Geometry: final body of the model. Coordinates: model frame, mm. A direction names the side the tool comes from. Round coordinates to 2 decimals unless told otherwise and drop trailing zeros. Loops run counter-clockwise (first coordinate to the right, second up) from the corner with the lowest first, then second, coordinate; pieces in that order, holes last. Notation, with made-up numbers: (19, -22) - (78, -22) arc R14 cw to (78, -13) - close; hole circle Ø10 at (4.25, 78.25). An arc over 180 degrees is marked (long way). Write item = value, one per line. Start each with the question number.
Item 1: Draft query along Z for faces 4 (the flat face through (0, 1, -27.403)), 5 (the cylindrical face through (-0.18, 4.02, 12.76)), 6 (the flat face through (-29.905, 4, 25)). Return one class per face: pulls with the +Z half, pulls with the -Z half, needs draft (parallel to the pull), parting line crosses it, or undercut.
Item 2: Section C-C (y = 1.05). Return loops of the section in (x, z), plus the area to 3 significant figures.
Item 3: Section A-A (x = 0). Return loops of the section in (y, z), plus the area to 3 significant figures.
Item 4: Section B-B (z = -22). Return loops of the section in (x, y).
Item 5: Section D-D (z = 9.5). Return loops of the section in (x, y).
Item 6: First-contact query: pin 1 (4 mm diameter, centred on x = -25.91, z = 24.6, fed in from -Y); pin 2 (1.1 mm diameter, centred on x = -29.5, y = 3, fed in from -Z); pin 3 (1.6 mm diameter, centred on x = -10, y = 0.5, fed in from +Z). Flat tips, straight axial feed; report the tip coordinate or a pass-through.
Item 7: Line query: line 1 (Z direction, x = 26, y = 3.45); line 2 (Z direction, x = 12, y = 3.1); line 3 (Z direction, x = -11, y = 4.9). Output: solid intervals per line, ascending. Write a range as from..to.
Item 8: Access query for faces 1 (the flat face through (-11.905, 5, -24)), 2 (the flat face through (0, 2, -33)), 3 (the flat face through (0, 2, 26)). Directions: +Z, -Z, +X, -X, +Y, -Y. A direction counts if a zero-diameter tool reaches every point of the face in a straight line with its end or side. Return the directions, or none.
from build123d import *

# Parameters (mm, degrees)
SKETCH1_W           = 60
SKETCH1_H           = 48
BOSS_EXTRUDE1_DEPTH = 2
BOSS_EXTRUDE2_DEPTH = 3.5
SKETCH3_W           = 6.52386431
SKETCH3_H           = 49
SKETCH3_W_2         = 6.523864309
CUT_EXTRUDE2_DEPTH  = 15
SKETCH4_W           = 24
SKETCH4_H           = 12
CUT_EXTRUDE3_DEPTH  = 1.5
SKETCH5_R           = 1.35
CUT_EXTRUDE4_DEPTH  = 3
SKETCH6_R           = 1.35
CUT_EXTRUDE5_DEPTH  = 3
SKETCH7_W           = 69.929961246
SKETCH7_H           = 12.314710156
SKETCH7_W_2         = 77.406749556
SKETCH7_H_2         = 16.199708004
CUT_EXTRUDE6_DEPTH  = 2
SKETCH8_R           = 1.6
CUT_EXTRUDE7_DEPTH  = 18
SKETCH9_W           = 6.597166155
SKETCH9_H           = 6.303958771
SKETCH9_W_2         = 5.93744954
SKETCH9_H_2         = 5.497638462
SKETCH9_W_3         = 7.769995694
SKETCH9_W_4         = 5.131129232
SKETCH9_H_3         = 5.204431078
SKETCH9_W_5         = 5.497638463
SKETCH9_H_4         = 5.0930957
SKETCH9_W_6         = 4.691318155
BOSS_EXTRUDE3_DEPTH = 3.5
SKETCH10_W          = 13.673673514
SKETCH10_H          = 2.686711401
SKETCH10_W_2        = 10.911645047
SKETCH10_H_2        = 3.141048784
SKETCH10_W_3        = 10.921694408
SKETCH10_H_3        = 3.054325349
SKETCH10_W_4        = 12
BOSS_EXTRUDE4_DEPTH = 3.5


with BuildPart() as part:
    # Sketch1 → Boss-Extrude1 (new body)
    with BuildSketch(Plane(origin=(0, 0, 0), x_dir=(1, 0, 0), z_dir=(0, 1, 0))):
        with Locations((0.094538135, 3.403372847)):
            Rectangle(SKETCH1_W, SKETCH1_H)
        with BuildLine():
            Line((-29.905461865, -20.596627153), (-29.905461865, -28.096627153))
            ThreePointArc((-29.905461865, -28.096627153), (-29.026782209, -30.217947496), (-26.905461865, -31.096627153))
            Line((-26.905461865, -31.096627153), (-24.905461865, -31.096627153))
            Line((-24.905461865, -31.096627153), (-24.905461865, -29.096627153))
            Line((-24.905461865, -29.096627153), (-14.905461865, -29.096627153))
            Line((-14.905461865, -29.096627153), (-14.905461865, -31.096627153))
            Line((-14.905461865, -31.096627153), (13.094538135, -31.096627153))
            Line((13.094538135, -31.096627153), (13.094538135, -29.096627153))
            Line((13.094538135, -29.096627153), (23.094538135, -29.096627153))
            Line((23.094538135, -29.096627153), (23.094538135, -31.096627153))
            Line((23.094538135, -31.096627153), (27.094538135, -31.096627153))
            ThreePointArc((27.094538135, -31.096627153), (29.215858478, -30.217947496), (30.094538135, -28.096627153))
            Line((30.094538135, -28.096627153), (30.094538135, -20.596627153))
            Line((30.094538135, -20.596627153), (-29.905461865, -20.596627153))
        make_face()
        with BuildLine():
            Line((30.094538135, 27.403372847), (30.094538135, 34.903372847))
            ThreePointArc((30.094538135, 34.903372847), (29.215858478, 37.024693191), (27.094538135, 37.903372847))
            Line((27.094538135, 37.903372847), (25.094538135, 37.903372847))
            Line((25.094538135, 37.903372847), (25.094538135, 35.903372847))
            Line((25.094538135, 35.903372847), (15.094538135, 35.903372847))
            Line((15.094538135, 35.903372847), (15.094538135, 37.903372847))
            Line((15.094538135, 37.903372847), (-12.905461865, 37.903372847))
            Line((-12.905461865, 37.903372847), (-12.905461865, 35.903372847))
            Line((-12.905461865, 35.903372847), (-22.905461865, 35.903372847))
            Line((-22.905461865, 35.903372847), (-22.905461865, 37.903372847))
            Line((-22.905461865, 37.903372847), (-26.905461865, 37.903372847))
            ThreePointArc((-26.905461865, 37.903372847), (-29.026782209, 37.024693191), (-29.905461865, 34.903372847))
            Line((-29.905461865, 34.903372847), (-29.905461865, 27.403372847))
            Line((-29.905461865, 27.403372847), (30.094538135, 27.403372847))
        make_face()
    extrude(amount=BOSS_EXTRUDE1_DEPTH)

    # Sketch2 → Boss-Extrude2 (add)
    with BuildSketch(Plane(origin=(0, 2, 0), x_dir=(1, 0, 0), z_dir=(0, 1, 0))):
        with BuildLine():
            Line((30.094538135, -11.096627153), (-29.905461865, -11.096627153))
            Line((-29.905461865, -11.096627153), (-29.905461865, -28.096627153))
            ThreePointArc((-29.905461865, -28.096627153), (-29.026782209, -30.217947496), (-26.905461865, -31.096627153))
            Line((-26.905461865, -31.096627153), (-24.905461865, -31.096627153))
            Line((-24.905461865, -31.096627153), (-24.905461865, -29.096627153))
            Line((-24.905461865, -29.096627153), (-14.905461865, -29.096627153))
            Line((-14.905461865, -29.096627153), (-14.905461865, -31.096627153))
            Line((-14.905461865, -31.096627153), (13.094538135, -31.096627153))
            Line((13.094538135, -31.096627153), (13.094538135, -29.096627153))
            Line((13.094538135, -29.096627153), (23.094538135, -29.096627153))
            Line((23.094538135, -29.096627153), (23.094538135, -31.096627153))
            Line((23.094538135, -31.096627153), (27.094538135, -31.096627153))
            ThreePointArc((27.094538135, -31.096627153), (29.215858478, -30.217947496), (30.094538135, -28.096627153))
            Line((30.094538135, -28.096627153), (30.094538135, -11.096627153))
        make_face()
        with BuildLine():
            Line((-29.905461865, 34.903372847), (-29.905461865, 17.903372847))
            Line((-29.905461865, 17.903372847), (30.094538135, 17.903372847))
            Line((30.094538135, 17.903372847), (30.094538135, 34.903372847))
            ThreePointArc((30.094538135, 34.903372847), (29.215858478, 37.024693191), (27.094538135, 37.903372847))
            Line((27.094538135, 37.903372847), (25.094538135, 37.903372847))
            Line((25.094538135, 37.903372847), (25.094538135, 35.903372847))
            Line((25.094538135, 35.903372847), (15.094538135, 35.903372847))
            Line((15.094538135, 35.903372847), (15.094538135, 37.903372847))
            Line((15.094538135, 37.903372847), (-12.905461865, 37.903372847))
            Line((-12.905461865, 37.903372847), (-12.905461865, 35.903372847))
            Line((-12.905461865, 35.903372847), (-22.905461865, 35.903372847))
            Line((-22.905461865, 35.903372847), (-22.905461865, 37.903372847))
            Line((-22.905461865, 37.903372847), (-26.905461865, 37.903372847))
            ThreePointArc((-26.905461865, 37.903372847), (-29.026782209, 37.024693191), (-29.905461865, 34.903372847))
        make_face()
    extrude(amount=BOSS_EXTRUDE2_DEPTH)

    # Sketch3 → Cut-Extrude2 (cut)
    with BuildSketch(Plane(origin=(0, 5.5, 0), x_dir=(1, 0, 0), z_dir=(0, 1, 0))):
        with Locations((-32.16739402, 3.403372847)):
            Rectangle(SKETCH3_W, SKETCH3_H)
        with Locations((32.35647029, 3.403372847)):
            Rectangle(SKETCH3_W_2, SKETCH3_H)
    extrude(amount=-CUT_EXTRUDE2_DEPTH, mode=Mode.SUBTRACT)

    # Sketch4 → Cut-Extrude3 (cut)
    with BuildSketch(Plane(origin=(0, 5.5, 0), x_dir=(1, 0, 0), z_dir=(0, 1, 0))):
        with Locations((0.094538135, 23.903372847)):
            Rectangle(SKETCH4_W, SKETCH4_H)
    extrude(amount=-CUT_EXTRUDE3_DEPTH, mode=Mode.SUBTRACT)

    # Sketch5 → Cut-Extrude4 (cut)
    with BuildSketch(Plane(origin=(0, 5.5, 0), x_dir=(1, 0, 0), z_dir=(0, 1, 0))):
        with Locations((0, -14.096627153)):
            Circle(SKETCH5_R)
    extrude(amount=-CUT_EXTRUDE4_DEPTH, mode=Mode.SUBTRACT)

    # Sketch6 → Cut-Extrude5 (cut)
    with BuildSketch(Plane(origin=(0, 5.5, 0), x_dir=(1, 0, 0), z_dir=(0, 1, 0))):
        with Locations((20.770286942, 25.903372847)):
            Circle(SKETCH6_R)
        with Locations((0, 31.903372847)):
            Circle(SKETCH6_R)
        with Locations((-20.187989902, 25.903372847)):
            Circle(SKETCH6_R)
        with Locations((-20.187989902, -19.096627153)):
            Circle(SKETCH6_R)
        with Locations((0, -25.096627153)):
            Circle(SKETCH6_R)
        with Locations((20.770286942, -19.096627153)):
            Circle(SKETCH6_R)
    extrude(amount=-CUT_EXTRUDE5_DEPTH, mode=Mode.SUBTRACT)

    # Sketch7 → Cut-Extrude6 (cut)
    with BuildSketch(Plane.XZ):
        with Locations((1.157414904, 26.753982231)):
            Rectangle(SKETCH7_W, SKETCH7_H)
        with Locations((2.037037058, -35.503226849)):
            Rectangle(SKETCH7_W_2, SKETCH7_H_2)
    extrude(amount=-CUT_EXTRUDE6_DEPTH, mode=Mode.SUBTRACT)

    # Sketch8 → Cut-Extrude7 (cut)
    with BuildSketch(Plane.XZ.offset(-2)):
        with Locations((-25.905461865, -31.403372847)):
            Circle(SKETCH8_R)
        with Locations((-9.905461865, -31.403372847)):
            Circle(SKETCH8_R)
        with Locations((10.094538135, -31.403372847)):
            Circle(SKETCH8_R)
        with Locations((26.094538135, -31.403372847)):
            Circle(SKETCH8_R)
        with Locations((26.094538135, 24.596627153)):
            Circle(SKETCH8_R)
        with Locations((10.094538135, 24.596627153)):
            Circle(SKETCH8_R)
        with Locations((-9.905461865, 24.596627153)):
            Circle(SKETCH8_R)
        with Locations((-25.905461865, 24.596627153)):
            Circle(SKETCH8_R)
    extrude(amount=-CUT_EXTRUDE7_DEPTH, mode=Mode.SUBTRACT)

    # Sketch9 → Boss-Extrude3 (add)
    with BuildSketch(Plane(origin=(0, 5.5, 0), x_dir=(1, 0, 0), z_dir=(0, 1, 0))):
        with Locations((-0.455225712, -25.037743467)):
            Rectangle(SKETCH9_W, SKETCH9_H)
        with Locations((20.399149524, -19.13694485)):
            Rectangle(SKETCH9_W_2, SKETCH9_H_2)
        with Locations((-21.272950024, -19.13694485)):
            Rectangle(SKETCH9_W_3, SKETCH9_H_2)
        with Locations((-20.759837101, 26.236897929)):
            Rectangle(SKETCH9_W_4, SKETCH9_H_3)
        with Locations((0.094538135, 32.449920697)):
            Rectangle(SKETCH9_W_5, SKETCH9_H_4)
        with Locations((20.362498601, 26.236897929)):
            Rectangle(SKETCH9_W_6, SKETCH9_H_3)
    extrude(amount=-BOSS_EXTRUDE3_DEPTH)

    # Sketch10 → Boss-Extrude4 (add)
    with BuildSketch(Plane.XZ.offset(-2)):
        with Locations((-18.068625108, 29.753271453)):
            Rectangle(SKETCH10_W, SKETCH10_H)
        with Locations((18.550360659, 29.526102761)):
            Rectangle(SKETCH10_W_2, SKETCH10_H_2)
        with Locations((-18.366309069, -36.376210173)):
            Rectangle(SKETCH10_W_3, SKETCH10_H_3)
        with Locations((19.094538135, -36.376210173)):
            Rectangle(SKETCH10_W_4, SKETCH10_H_3)
    extrude(amount=-BOSS_EXTRUDE4_DEPTH)


solid = part.part
Taken from the geometry:
q1.face_4 = pulls with the -Z half
q1.face_5 = undercut
q1.face_6 = needs draft
q2.outline = (-28.91, -27.4) - (29.09, -27.4) - (29.09, 20.6) - (-28.91, 20.6) - close
q2.area = 2,780 mm^2
q3.outline = (0, -27.4) - (2, -27.4) - (2, -37.9) - (5.5, -37.9) - (5.5, -29.9) - (4, -29.9) - (4, -17.9) - (2, -17.9) - (2, 11.1) - (5.5, 11.1) - (5.5, 12.75) - (2.5, 12.75) - (2.5, 15.45) - (5.5, 15.45) - (5.5, 31.1) - (2, 31.1) - (2, 20.6) - (0, 20.6) - close
q3.area = 210 mm^2
q4.outline = (-28.91, 0) - (29.09, 0) - (29.09, 5.5) - (12.09, 5.5) - (12.09, 4) - (-11.91, 4) - (-11.91, 5.5) - (-28.91, 5.5) - close
q5.outline = (-28.91, 0) - (29.09, 0) - (29.09, 2) - (-28.91, 2) - close
q6.pin_1 = 2
q6.pin_2 = -37.1
q6.pin_3 = 20.6
q7.line_1 = -37.9..-33, -29.81..-17.9, 11.1..23, 26.19..31.1
q7.line_2 = -37.9..-17.9, 11.1..31.1
q7.line_3 = -37.9..-32.57, -30.24..-29.9, 11.1..23.43, 25.76..31.1
q8.face_1 = +Y
q8.face_2 = -Z, +X, -X, -Y
q8.face_3 = +Z, +X, -X, -Y
